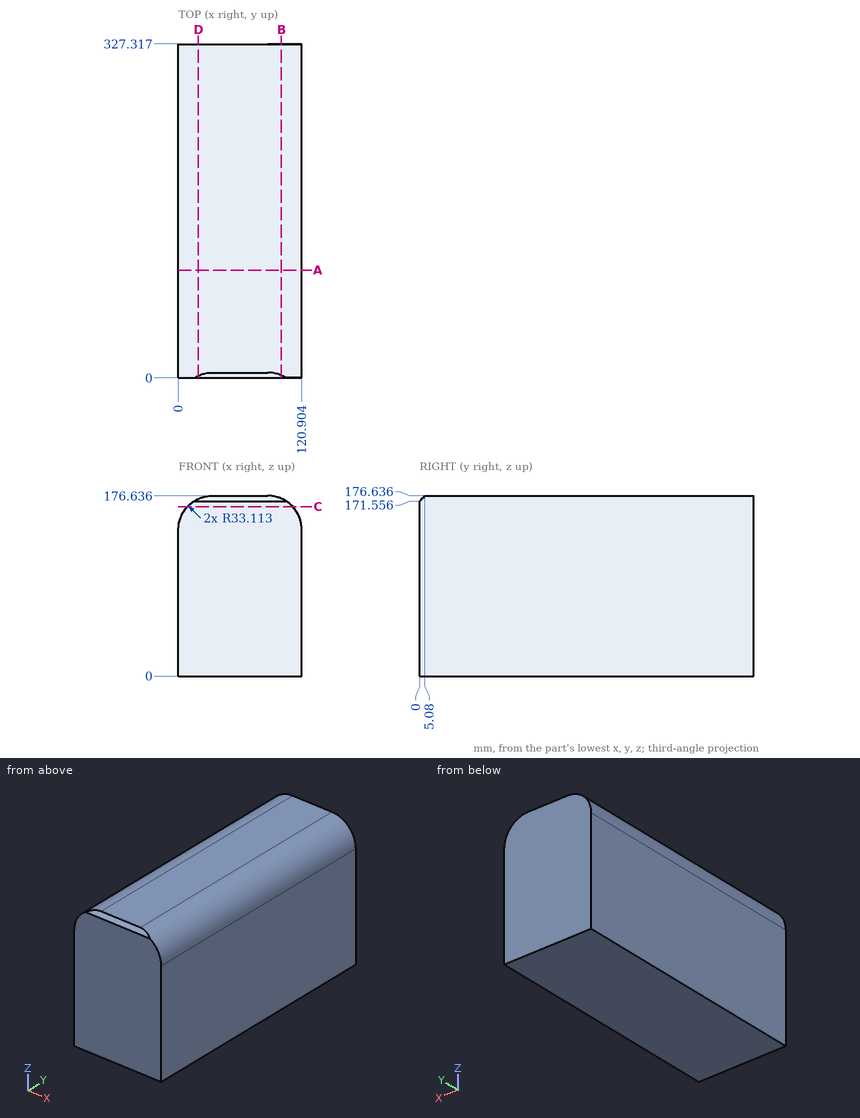
Input: dimensioned drawing with shaded views. Units: mm. Origin: part minimum x, y, z. Coordinates: 2 decimals unless noted, no trailing zeros. Loops run counter-clockwise (first coordinate to the right, second up) from the corner with the lowest first, then second, coordinate; pieces in that order, holes last. Notation, with made-up numbers: M 34,-17.75 L 88,-17.75 A13 ccw 88,-11.75 Z; hole C 88,59 d2. An arc over 180 degrees is marked long. One line per item, written item: value.
(1) Line query: line 1 along Z through (x, y) = (110.5, 200); line 2 along X through (y, z) = (188.5, 169) (1 decimal); line 3 along Z through (x, y) = (107.5, 169). Output: solid intervals per line, ascending. Write a range as from..to.
Filled in:
line 1: 0..167.62
line 2: 12..108.9
line 3: 0..170.13
(2) Section C-C (z = 166). Output: boundary loops of the cut face in (x, y).
Filled in:
outline: M 8.8,0 L 112.11,0 L 112.11,327.32 L 8.8,327.32 Z
(3) Pin query (flat end, axial travel): pin 1 (1.5 mm diameter, centred on x = 23, y = 78, fed in from -Z). Return the tip coordinate at first contact, or that it passes through.
Filled in:
pin 1: z = 0
(4) Section A-A (y = 105.5). Output: boundary loops of the cut face in (x, z), and give its area (3 significant figures).
Filled in:
outline: M 0,0 L 120.9,0 L 120.9,143.52 A33.11 ccw 87.79,176.64 L 33.11,176.64 A33.11 ccw 0,143.52 Z
area: 20,900 mm^2
(5) Section B-B (x = 101). Output: boundary loops of the cut face in (y, z).
Filled in:
outline: M 0,0 L 327.32,0 L 327.32,173.89 L 2.33,173.89 L 0,171.56 Z
(6) Section D-D (x = 19.5). Output: boundary loops of the cut face in (y, z), and give its area (3 significant figures).
Filled in:
outline: M 0,0 L 327.32,0 L 327.32,173.71 L 2.15,173.71 L 0,171.56 Z
area: 56,900 mm^2
